```python
from build123d import *

# Parameters (mm, degrees)
F0_R     = 11.1125
F1_DEPTH = 41.275
F2_R     = 6.35
F3_DEPTH = 82.55
F4_R     = 1.778
F5_DEPTH = 11.1125
F6_R     = 1.778
F7_DEPTH = 11.1125


with BuildPart() as f1:
    # F0 (on Top) → F1 (new body, symmetric)
    with BuildSketch(Plane.XY):
        Circle(F0_R)
    extrude(amount=F1_DEPTH, both=True)

    # F2 (on face) → F3 (cut, through all)
    with BuildSketch(Plane.XY.offset(41.275)):
        Circle(F2_R)
    extrude(amount=-F3_DEPTH, mode=Mode.SUBTRACT)

    # F4 (on Right) → F5 (cut, symmetric)
    with BuildSketch(Plane.YZ):
        with Locations((0, 10.922)):
            Circle(F4_R)
    extrude(amount=F5_DEPTH, both=True, mode=Mode.SUBTRACT)

    # F6 (on Right) → F7 (cut, symmetric)
    with BuildSketch(Plane.YZ):
        with Locations((0, -13.97)):
            Circle(F6_R)
    extrude(amount=F7_DEPTH, both=True, mode=Mode.SUBTRACT)


solid = f1.part
```
Here's how the part is built. I have some questions about the finished solid (model axes, mm). Give positions to 0.01 mm unless a question says otherwise; leave off trailing zeros. Order: outer loops, then holes, each group sorted by start corner. A loop starts at its lowest first (then second) coordinate and runs counter-clockwise, first axis right, second up. Notation, with made-up numbers: (-6, 17) - (21, 17) arc R18 ccw to (21, 21) - close; hole circle Ø11 at (76, 15.5). An arc over 180 degrees is marked (long way). Answer as a JSON object with one key per item and string values. Group by question number.
Item 1: For P1, Ø6, axis at y = -6.5, z = -22.5, coming from the -X side; P2, Ø11.5, axis at x = 0, y = 0, coming from the -Z side; P3, Ø6, axis at y = -8, z = -16.5, coming from the -X side; P4, Ø5.5, axis at y = 0, z = -13.97, coming from the +X side, each with a flat end and sliding along its axis, tell me the tip position at first contact or that it passes through.
Item 2: Please list where these lines run through material, in increasing order: probe 1 along Z at (x, y) = (7.9, 0) (3 decimals); probe 2 along Y at (x, z) = (0, 20.5).
Item 3: If we section it at D-D on x = 7.5: Please give me the cut outline in (y, z) (3 decimals), and give its area (3 significant figures).
Item 4: If we section it at A-A on y = 0: Give the number of separate pieces and of enclosed holes in the cut face, and give its area (3 significant figures).
Item 5: If we mould it in two halves opening along X, with no side actions, what happens to faces 1 (the cylindrical face through (10.6, 3.34, 0.58)), 2 (the cylindrical face through (6.057, 1.907, 0.578)), 3 (the cylindrical face through (8.639, -0.231, -12.207))? For each: pulls with the +X half, pulls with the -X half, needs draft (parallel to the pull), parting line crosses it, or undercut.
Result set:
{
 "1": {"P1": "x = -10.55", "P2": "through", "P3": "x = -9.92", "P4": "x = 11.11"},
 "2": {"probe 1": "-41.275 to -15.748, -12.192 to 9.144, 12.7 to 41.275", "probe 2": "-11.11 to -6.35, 6.35 to 11.11"},
 "3": {"outline": "(-8.2, -41.275) - (8.2, -41.275) - (8.2, 41.275) - (-8.2, 41.275) - close; hole circle Ø3.556 at (0, -13.97); hole circle Ø3.556 at (0, 10.922)", "area": "1,330 mm²"},
 "4": {"separate pieces": "6", "enclosed holes": "0", "area": "719 mm²"},
 "5": {"face 1": "parting line crosses it", "face 2": "undercut", "face 3": "needs draft"}
}
